Answer from the drawing. Dimensions are ordinates in mm from the lowest x, y and z of the part. A direction names the side the tool comes from. Give positions to 0.01 mm unless a question says otherwise; leave off trailing zeros. Loops run counter-clockwise (first coordinate to the right, second up) from the corner with the lowest first, then second, coordinate; pieces in that order, holes last. Notation, with made-up numbers: (45, 0) -> (53, 0) arc R22 ccw to (53, 35) -> close; hole circle Ø8 at (74.5, 66.5). An arc over 180 degrees is marked (long way). Return JSON: item names as keys, results as strings. Group by question number.
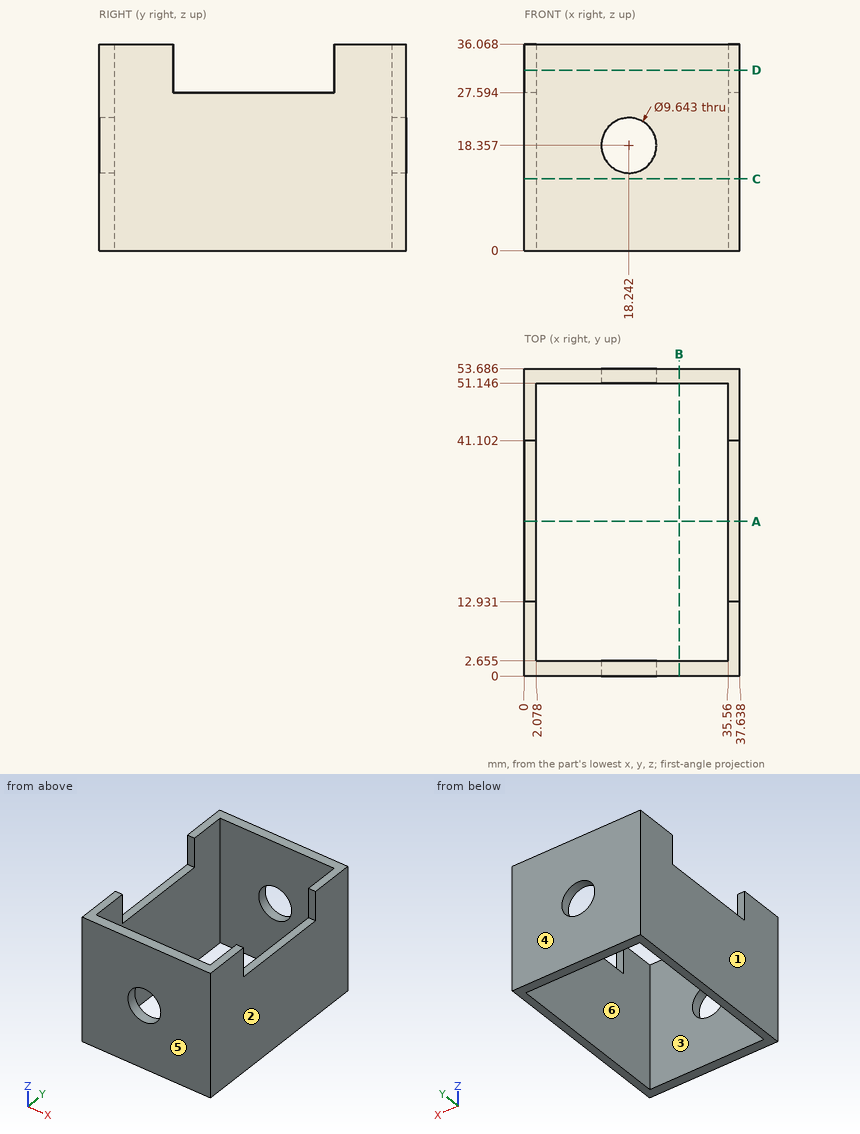
1. Section D-D on z = 31.5 is taken. Determine the outline of the cut face in (x, y) (1 decimal).
2. Section A-A on y = 27 is taken. Determine the outline of the cut face in (x, z), then the cut area to 3 significant figures.
3. Which of the six approach directions +Z, -Z, +X, -X, +Y, -Y give full straight-line access (tool end or side, diameter ignored) to the marked faces 5 and 6?
4. Straight lines are drawn through the part: line 1 (X direction, y = 10, z = 31); line 2 (Y direction, x = 31, z = 9.5) (1 decimal); line 3 (Z direction, x = 2, y = 29.5). For each, find the intervals that lie inside material, in ascending order. Write a range as from..to.
5. Section B-B on x = 27 is taken. Determine the outline of the cut face in (y, z) (1 decimal).
6. Section C-C on z = 12.5 is taken. Determine the outline of the cut face in (x, y) (1 decimal).
7. Determine the mould class of the marked faces 1, 2, 3 and 4 for opening direction X: pulls with the +X half, pulls with the -X half, needs draft (parallel to the pull), parting line crosses it, or undercut.
8. Flat-ended cylindrical pins translate along their axes: pin 1 Ø6 at (x, y) = (6.5, 21.5) entering from -Z; pin 2 Ø2.5 at (x, y) = (37, 33) entering from +Z. Find the tip coordinate at first contact, or state that the pin passes through.
Completed:
{
 "1": {"outline": "(0, 0) -> (37.6, 0) -> (37.6, 12.9) -> (35.6, 12.9) -> (35.6, 2.7) -> (2.1, 2.7) -> (2.1, 12.9) -> (0, 12.9) -> close; (0, 41.1) -> (2.1, 41.1) -> (2.1, 51.1) -> (35.6, 51.1) -> (35.6, 41.1) -> (37.6, 41.1) -> (37.6, 53.7) -> (0, 53.7) -> close"},
 "2": {"outline": "(0, 0) -> (2.08, 0) -> (2.08, 27.59) -> (0, 27.59) -> close; (35.56, 0) -> (37.64, 0) -> (37.64, 27.59) -> (35.56, 27.59) -> close", "area": "115 mm²"},
 "3": {"face 5": "+Z, -Z, +X, -X, -Y", "face 6": "+Z, -Z"},
 "4": {"line 1": "x = 0..2.08, 35.56..37.64", "line 2": "y = 0..2.7, 51.1..53.7", "line 3": "z = 0..27.59"},
 "5": {"outline": "(0, 0) -> (2.7, 0) -> (2.7, 36.1) -> (0, 36.1) -> close; (51.1, 0) -> (53.7, 0) -> (53.7, 36.1) -> (51.1, 36.1) -> close"},
 "6": {"outline": "(0, 0) -> (37.6, 0) -> (37.6, 53.7) -> (0, 53.7) -> close; hole (2.1, 2.7) -> (35.6, 2.7) -> (35.6, 51.1) -> (2.1, 51.1) -> close"},
 "7": {"face 1": "pulls with the -X half", "face 2": "pulls with the +X half", "face 3": "undercut", "face 4": "needs draft"},
 "8": {"pin 1": "passes through", "pin 2": "stops at z = 27.59"}
}
